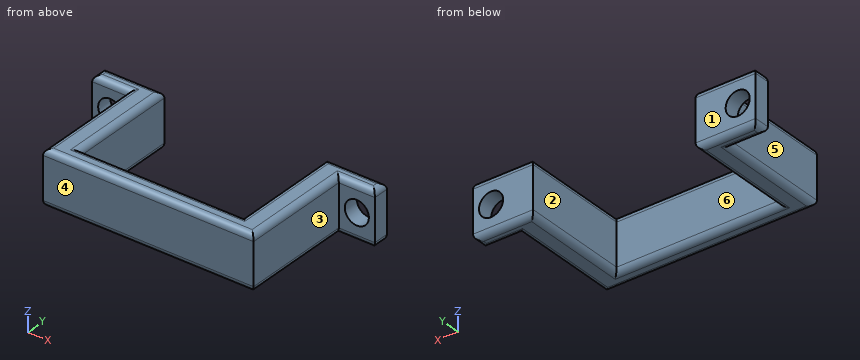
from build123d import *

# Parameters (mm, degrees)
BOSS_EXTRUDE1_DEPTH = 9
SKETCH2_R           = 2
CUT_EXTRUDE1_DEPTH  = 9
FILLET1_R           = 1


with BuildPart() as part:
    # Sketch1 → Boss-Extrude1 (new body)
    with BuildSketch(Plane.XY):
        Polygon((0, 0), (10, 0), (10, -18), (37, -18), (37, 0), (47, 0), (47, -2.614456703), (41, -2.614456703), (41, -21), (6, -21), (6, -2.614456703), (0, -2.614456703), align=None)
    extrude(amount=BOSS_EXTRUDE1_DEPTH)

    # Sketch2 → Cut-Extrude1 (cut)
    with BuildSketch(Plane.XZ.offset(2.614456703)):
        with Locations((3, 4.5)):
            Circle(SKETCH2_R)
    cut_extrude1 = extrude(amount=-CUT_EXTRUDE1_DEPTH, mode=Mode.SUBTRACT)

    # Mirror1: Cut-Extrude1 across plane
    add(cut_extrude1.mirror(Plane(origin=(23.5, 0, 0), x_dir=(0, 0, 1), z_dir=(1, 0, 0))), mode=Mode.SUBTRACT)

    # Fillet1
    fillet1_edges = [part.edges().sort_by_distance(p)[0] for p in [
        (5, 0, 0),
        (10, -9, 0),
        (6, -11.807228352, 9),
        (23.5, -18, 0),
        (37, -9, 0),
        (42, 0, 0),
        (47, -1.307228352, 0),
        (44, -2.614456703, 0),
        (41, -11.807228352, 0),
        (23.5, -21, 0),
        (6, -11.807228352, 0),
        (3, -2.614456703, 0),
        (0, -1.307228352, 0),
        (23.5, -21, 9),
        (41, -11.807228352, 9),
        (44, -2.614456703, 9),
        (47, -1.307228352, 9),
        (42, 0, 9),
        (37, -9, 9),
        (23.5, -18, 9),
        (10, -9, 9),
        (5, 0, 9),
        (0, -1.307228352, 9),
        (3, -2.614456703, 9),
    ]]
    fillet(fillet1_edges, radius=FILLET1_R)


solid = part.part
Verification items for the finished model (mm, model axes). Face numbers are marked on the shaded views. A direction names the side the tool comes from. Round coordinates to 2 decimals unless told otherwise and drop trailing zeros. Loops run counter-clockwise (first coordinate to the right, second up) from the corner with the lowest first, then second, coordinate; pieces in that order, holes last. Notation, with made-up numbers: (30.25, 89.25) - (50.25, 89.25) arc R15 ccw to (50.25, 103.25) - close; hole circle Ø11 at (-40, 62.5). An arc over 180 degrees is marked (long way). Answer in a Markdown table with one row per item. Add a question column.
Q1. Section check C-C on x = 44. Enter the section's corners in (y, z).
Q2. Tool access check on the marked faces 4, 5 and 6. Record the directions out of +Z, -Z, +X, -X, +Y, -Y that give a thin tool (end or side, any length) a straight path to the whole face; none if there is none.
Q3. Section check A-A on y = -4.75. Enter the section's corners in (x, z).
Q4. Section check B-B on z = 4.5. Enter the section's corners in (x, y), plus the area to 3 significant figures.
Q5. Section check D-D on x = 14.5. Enter the section's corners in (y, z).
Q6. Release check for a two-part mould opening along X. For the marked faces 1, 2 and 3 record: pulls with the +X half, pulls with the -X half, needs draft (parallel to the pull), parting line crosses it, or undercut.
Q7. Material ranges on line 1 (Z direction, x = 3, y = -1.15); line 2 (X direction, y = -16.25, z = 6.75); line 3 (X direction, y = -1, z = 2.25), recorded low to high.
Q8. Gauge pin test, flat ends, axial feed: pin 1 (2 mm diameter, centred on y = -11.5, z = 6, fed in from +X); pin 2 (2 mm diameter, centred on y = -7, z = 5, fed in from -X); pin 3 (2.5 mm diameter, centred on x = 3, z = 4.5, fed in from -Y). Record the tip position at first contact, or that the pin passes through.
Found:
| question | item | result |
|---|---|---|
| 1 | outline | (-2.61, 1) arc R1 ccw to (-1.61, 0) - (-1, 0) arc R1 ccw to (0, 1) - (0, 2.5) - (-2.61, 2.5) - close; (-2.61, 6.5) - (0, 6.5) - (0, 8) arc R1 ccw to (-1, 9) - (-1.61, 9) arc R1 ccw to (-2.61, 8) - close |
| 2 | face 4 | +Z, -Z, +X, -X, -Y |
| 2 | face 5 | +Z, -Z, -X, -Y |
| 2 | face 6 | +Z, -Z, +Y |
| 3 | outline | (6, 1) arc R1 ccw to (7, 0) - (9, 0) arc R1 ccw to (10, 1) - (10, 8) arc R1 ccw to (9, 9) - (7, 9) arc R1 ccw to (6, 8) - close; (37, 1) arc R1 ccw to (38, 0) - (40, 0) arc R1 ccw to (41, 1) - (41, 8) arc R1 ccw to (40, 9) - (38, 9) arc R1 ccw to (37, 8) - close |
| 4 | outline | (0, -2.61) - (1, -2.61) - (1, 0) - (0, 0) - close; (5, -2.61) - (6, -2.61) - (6, -21) - (41, -21) - (41, -2.61) - (42, -2.61) - (42, 0) - (37, 0) - (37, -18) - (10, -18) - (10, 0) - (5, 0) - close; (46, -2.61) - (47, -2.61) - (47, 0) - (46, 0) - close |
| 4 | area | 259 mm² |
| 5 | outline | (-21, 1) arc R1 ccw to (-20, 0) - (-19, 0) arc R1 ccw to (-18, 1) - (-18, 8) arc R1 ccw to (-19, 9) - (-20, 9) arc R1 ccw to (-21, 8) - close |
| 6 | face 1 | needs draft |
| 6 | face 2 | undercut |
| 6 | face 3 | pulls with the +X half |
| 7 | line 1 | z = 0 to 2.5, 6.5 to 9 |
| 7 | line 2 | x = 6 to 10, 37 to 41 |
| 7 | line 3 | x = 0 to 10, 37 to 47 |
| 8 | pin 1 | stops at x = 41 |
| 8 | pin 2 | stops at x = 6 |
| 8 | pin 3 | passes through |
